Geometry: final body of the model. Coordinates: model frame, mm. Coordinates: 2 decimals unless noted, no trailing zeros. Write each loop counter-clockwise with the first axis right and the second up, starting at its lowest first coordinate (ties: lowest second). Pieces come first, ordered by that corner, then holes. Notation, with made-up numbers: (-35.5, 12.5) -> (6.5, 12.5) arc R24 ccw to (6.5, 26.5) -> close; hole circle Ø2 at (38, 63). An arc over 180 degrees is marked (long way). One line per item, written item: value.
```python
from build123d import *

# Parameters (mm, degrees)
F1_DEPTH = 3.7


with BuildPart() as f1:
    # F0 (on Front) → F1 (new body)
    with BuildSketch(Plane.XZ):
        with BuildLine():
            Line((0, 10.6), (0, 11.6))
            ThreePointArc((0, 11.6), (-5.857057, 9.433365), (-8.894091, 3.976641))
            Line((-8.894091, 3.976641), (-9.879779, -0.045725))
            Line((-9.879779, -0.045725), (-10.462536, 0.097081))
            Line((-10.462536, 0.097081), (-10.55774, -0.291424))
            Line((-10.55774, -0.291424), (-9.77304, -2.131056))
            Line((-9.77304, -2.131056), (-9.384535, -2.22626))
            Line((-9.384535, -2.22626), (-9.104897, -1.085122))
            Line((-9.104897, -1.085122), (-7.912193, 3.782031))
            ThreePointArc((-7.912193, 3.782031), (-5.222248, 8.660373), (0, 10.6))
        make_face()
        with BuildLine():
            ThreePointArc((8.894091, 3.976641), (5.857057, 9.433365), (0, 11.6))
            Line((0, 11.6), (0, 10.6))
            ThreePointArc((0, 10.6), (5.222248, 8.660373), (7.912193, 3.782031))
            Line((7.912193, 3.782031), (9.104897, -1.085122))
            Line((9.104897, -1.085122), (9.384535, -2.22626))
            Line((9.384535, -2.22626), (9.77304, -2.131056))
            Line((9.77304, -2.131056), (10.55774, -0.291424))
            Line((10.55774, -0.291424), (10.462536, 0.097081))
            Line((10.462536, 0.097081), (9.879779, -0.045725))
            Line((9.879779, -0.045725), (8.894091, 3.976641))
        make_face()
    extrude(amount=F1_DEPTH)


solid = f1.part
```
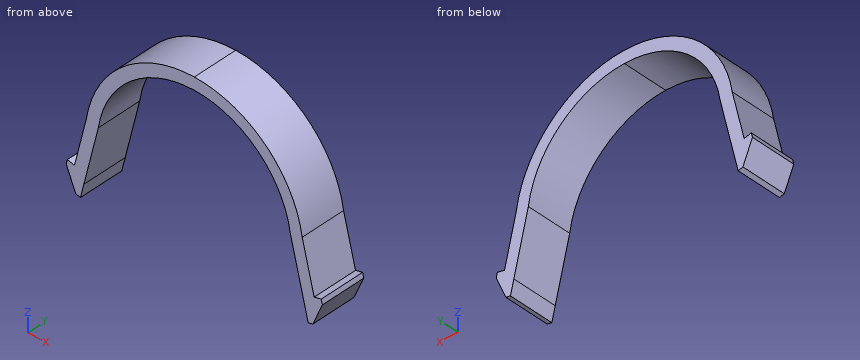
(1) Section B-B (z = 7.75). Return the cut outline in (x, y).
Responses:
outline: (-7.38, -3.7) -> (-6.12, -3.7) -> (-6.12, 0) -> (-7.38, 0) -> close; (6.12, -3.7) -> (7.38, -3.7) -> (7.38, 0) -> (6.12, 0) -> close
(2) First-contact query: pin 1 (1.5 mm diameter, centred on y = -2, z = 4.5, fed in from +X). Flat tip, straight axial feed; report the tip coordinate or a pass-through.
Responses:
pin 1: stops at x = 8.95
(3) Section A-A (y = -3.1). Return the cut outline in (x, z).
Responses:
outline: (-10.56, -0.29) -> (-9.77, -2.13) -> (-9.38, -2.23) -> (-9.1, -1.09) -> (-7.91, 3.78) arc R8 cw to (0, 10.6) arc R8 cw to (7.91, 3.78) -> (9.1, -1.09) -> (9.38, -2.23) -> (9.77, -2.13) -> (10.56, -0.29) -> (10.46, 0.1) -> (9.88, -0.05) -> (8.89, 3.98) arc R9 ccw to (0, 11.6) arc R9 ccw to (-8.89, 3.98) -> (-9.88, -0.05) -> (-10.46, 0.1) -> close
(4) Section D-D (x = -3.25). Return the cut outline in (y, z).
Responses:
outline: (-3.7, 9.91) -> (0, 9.91) -> (0, 10.99) -> (-3.7, 10.99) -> close
(5) Line query: line 1 (X direction, y = -3.1, z = 4.5); line 2 (X direction, y = -2.55, z = 8); line 3 (Z direction, x = -3.75, y = -0.55). Output: solid intervals per line, ascending. Write a range as [from, to].
Responses:
line 1: x = [-8.8, -7.77], [7.77, 8.8]
line 2: x = [-7.2, -5.9], [5.9, 7.2]
line 3: z = [9.67, 10.78]
(6) Section C-C (z = -0.75). Return the cut outline in (x, y), then the cut area to 3 significant figures.
Responses:
outline: (-10.36, -3.7) -> (-9.02, -3.7) -> (-9.02, 0) -> (-10.36, 0) -> close; (9.02, -3.7) -> (10.36, -3.7) -> (10.36, 0) -> (9.02, 0) -> close
area: 9.91 mm2
